Source: CAD feature listing. Evaluate the final solid. Frame: model axes, mm. Give positions to 0.01 mm unless a question says otherwise; leave off trailing zeros. Loops run counter-clockwise (first coordinate to the right, second up) from the corner with the lowest first, then second, coordinate; pieces in that order, holes last. Notation, with made-up numbers: M -17.5,-27.5 L -6.5,-27.5 A23 cw -6.5,-16.5 Z; hole C 72.25,45.5 d11. An arc over 180 degrees is marked long. Put each result on its own line as item: value.
Autodesk Inventor part; units mm, degrees
ref_plane "YZ Plane" through (0, 0, 0) normal (1, 0, 0) x (0, 1, 0)
ref_plane "XZ Plane" through (0, 0, 0) normal (0, 1, 0) x (-1, 0, 0)
ref_plane "XY Plane" through (0, 0, 0) normal (0, 0, 1) x (1, 0, 0)
sketch "Sketch1" plane through (0, 0, 0) normal (0, 0, 1) x (1, 0, 0)
  line L0 (0, 0) -> (0, 485)
  line L1 (-175, 485) -> (175, 485)
  circle A0 centre (0, 120) radius 62.5
  circle A1 centre (0, 120) radius 120
  line L2 (-175, 485) -> (-175, 288.2777)
  line L3 (-175, 288.2777) -> (-115.0584, 85.9182)
  line L4 (175, 485) -> (175, 288.2777)
  line L5 (175, 288.2777) -> (115.0584, 85.9182)
  dimension "d0" = 485
  dimension "d1" = 350
  dimension "d2" = 125
  dimension "d4" = 196.7223
  dimension "d16" = 33
  dimension "d17" = 240
extrude "Plate1" add sketch "Sketch1" along normal blind 10 contours A1 L0 A0 | L0 A0 A1 | L3 L2 L1 L0 A1 | A1 L0 L1 L4 L5
sketch "Sketch2" plane through (-175, 476.3397, 5) normal (0, 0.866, -0.5) x (-1, 0, 0)
  line L0 (-350, 0) -> (0, 0)
  line L1 (0, 0) -> (0, 40)
  line L2 (0, 40) -> (-350, 40)
  line L3 (-350, 40) -> (-350, 0)
equation "\"d2\" = back_steel_circle_проходной_диаметр"
equation "\"d5\" = Thickness"
equation "\"BendReliefDepth\" = 0.5 * Thickness"
properties part number "NVPH-301 back side"
1. Section query A-A (x = 0). Output: boundary loops of the cut face in (y, z).
Found:
outline: M 0,0 L 57.5,0 L 57.5,10 L 0,10 Z; M 182.5,0 L 485,0 L 485,10 L 182.5,10 Z
2. Contact query for flat-ended pins moving along their axis: P1, Ø5, axis at x = -76.5, z = 1.5, coming from the -Y side; P2, Ø6, axis at x = 40, z = 8.5, coming from the -Y side. Output: stop coordinate, or through.
Found:
P1: y = 25.53
P2: y = 5.85
3. Section query C-C (y = 120). Output: boundary loops of the cut face in (x, z).
Found:
outline: M -125.15,0 L -62.5,0 L -62.5,10 L -125.15,10 Z; M 62.5,0 L 125.15,0 L 125.15,10 L 62.5,10 Z
4. Section query D-D (x = 89). Output: boundary loops of the cut face in (y, z).
Found:
outline: M 39.51,0 L 485,0 L 485,10 L 39.51,10 Z
5. Section query B-B (z = 3.5). Output: boundary loops of the cut face in (x, y).
Found:
outline: M -175,288.28 L -115.06,85.92 A120 ccw 115.06,85.92 L 175,288.28 L 175,485 L -175,485 Z; hole C 0,120 d125
6. Material intervals for line 1 (Y direction, x = 0, z = 5.5); line 2 (X direction, y = 120, z = 7.25); line 3 (X direction, y = 125.5, z = 3.5), sorted ascending. Write a range as from..to.
Found:
line 1: 0..57.5, 182.5..485
line 2: -125.15..-62.5, 62.5..125.15
line 3: -126.78..-62.26, 62.26..126.78
7. Draft query along Y for faces 1 (the flat face through (-2, 300, 0)), 2 (the flat face through (-145.449, 188.514, 4.93)), 3 (the cylindrical face through (-13.549, 181.014, 4.93)). Return one class per face: pulls with the +Y half, pulls with the -Y half, needs draft (parallel to the pull), parting line crosses it, or undercut.
Found:
face 1: needs draft
face 2: pulls with the -Y half
face 3: undercut
